Could you check a few things on this drawing? It's one solid part, dimensions in mm from its lowest x, y, z. A direction names the side the tool comes from. Coordinates: 2 decimals unless noted, no trailing zeros. Loops run counter-clockwise (first coordinate to the right, second up) from the corner with the lowest first, then second, coordinate; pieces in that order, holes last. Notation, with made-up numbers: (45, 53) -> (94, 53) arc R14 ccw to (94, 79) -> close; hole circle Ø4 at (-6.5, 53.25). An arc over 180 degrees is marked (long way). One line per question, with ' | ' between items. Start each with the question number.
(1) Suppose I cut it at A-A (x = 7.5). Please give me the cut outline in (y, z).
(2) If I drill on line 1 along Y through (x, z) = (1.5, 11.5); line 2 along Z through (x, y) = (7.5, 3.5); line 3 along X through (y, z) = (0.75, 7.75), over which ranges is the centre line in solid material (lowest first)?
(3) I'm going to push flat-ended pins straight in: pin 1 Ø1 at (x, z) = (7, 8) entering from -Y; pin 2 Ø1 at (y, z) = (4.5, 7.5) entering from -X; pin 3 Ø1.5 at (y, z) = (6.5, 12) entering from +X; pin 4 Ø1 at (y, z) = (5, 4.5) entering from +X. Where does each tip first touch, or does it pass through?
(4) Suppose I cut it at B-B (z = 7.5). Please give me the cut outline in (x, y), plus the area to 3 significant figures.
(5) Suppose I cut it at C-C (y = 5.5). Please give me the cut outline in (x, z), plus the area to 3 significant figures.
(6) Suppose I cut it at D-D (z = 2.25). Please give me the cut outline in (x, y).
(7) Which directions (+Z, -Z, +X, -X, +Y, -Y) give clear straight access to the entire face, cutting with the end or side of a thin tool? Please do the marked faces 4 and 5.
(8) If we mould it in two halves opening along X, with no side actions, what happens to the marked faces 1, 2 and 3? For each: pulls with the +X half, pulls with the -X half, needs draft (parallel to the pull), parting line crosses it, or undercut.
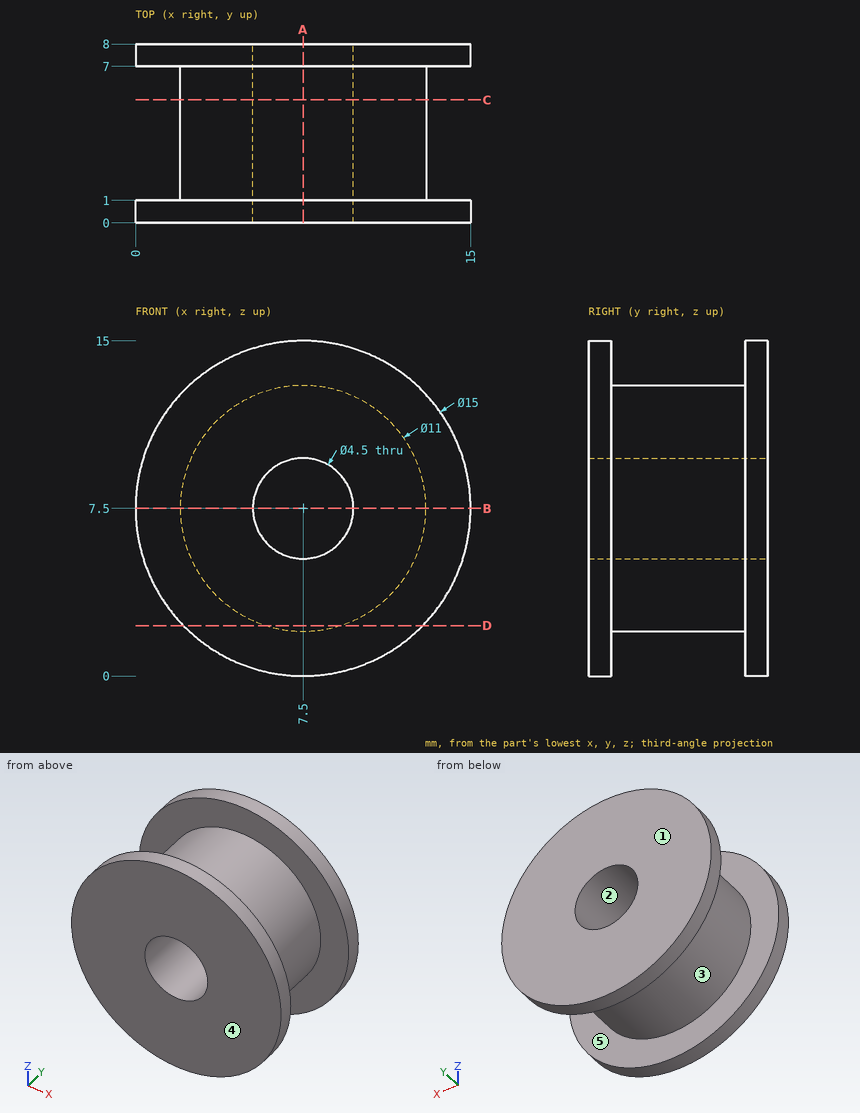
Checks:
1) outline: (0, 0) -> (1, 0) -> (1, 2) -> (7, 2) -> (7, 0) -> (8, 0) -> (8, 5.25) -> (0, 5.25) -> close; (0, 9.75) -> (8, 9.75) -> (8, 15) -> (7, 15) -> (7, 13) -> (1, 13) -> (1, 15) -> (0, 15) -> close
2) line 1: y = 0 to 1, 7 to 8 | line 2: z = 2 to 5.25, 9.75 to 13 | line 3: x = 0 to 5.26, 9.74 to 15
3) pin 1: passes through | pin 2: stops at x = 2 | pin 3: stops at x = 13.88 | pin 4: stops at x = 12.4
4) outline: (0, 0) -> (5.25, 0) -> (5.25, 8) -> (0, 8) -> (0, 7) -> (2, 7) -> (2, 1) -> (0, 1) -> close; (9.75, 0) -> (15, 0) -> (15, 1) -> (13, 1) -> (13, 7) -> (15, 7) -> (15, 8) -> (9.75, 8) -> close | area: 60.0 mm^2
5) outline: circle Ø11 at (7.5, 7.5); hole circle Ø4.5 at (7.5, 7.5) | area: 79.1 mm^2
6) outline: (2.14, 0) -> (12.86, 0) -> (12.86, 1) -> (9.14, 1) -> (9.14, 7) -> (12.86, 7) -> (12.86, 8) -> (2.14, 8) -> (2.14, 7) -> (5.86, 7) -> (5.86, 1) -> (2.14, 1) -> close
7) face 4: +Z, -Z, +X, -X, -Y | face 5: none
8) face 1: needs draft | face 2: undercut | face 3: parting line crosses it
